Check sheet for the modelled part. Datum: model origin and axes. Units: mm. A direction names the side the tool comes from. Round coordinates to 2 decimals unless told otherwise and drop trailing zeros. Loops run counter-clockwise (first coordinate to the right, second up) from the corner with the lowest first, then second, coordinate; pieces in that order, holes last. Notation, with made-up numbers: M -36.5,-32 L 17.5,-32 A26 cw 17.5,-13 Z; hole C -34.75,-10 d9. An arc over 180 degrees is marked long. Write item = value, one per line. Start each with the question number.
(1) Cross-section at B-B on x = 0.55. Record the boundary of the cut face in (y, z).
(2) Set-up check for faces 5 (the face through (2, -5, -22)), 6 (the face through (4, 0, -18)): record each of +Z, -Z, +X, -X, +Y, -Y from which the full face is reachable in a straight line by a thin tool's end or side.
(3) Cross-section at D-D on x = 3.95. Record the boundary of the cut face in (y, z) (3 decimals).
(4) Cross-section at C-C on z = -11.5. Record the boundary of the cut face in (x, y).
(5) Cross-section at A-A on y = -7.25. Record the boundary of the cut face in (x, z).
(6) Go/stop test with flat-tipped pins: P1, Ø1, axis at x = 1, z = -5.5, coming from the +Y side; P2, Ø1.5, axis at x = 2.5, y = -8, coming from the +Z side; P3, Ø3, axis at x = 1.5, y = -10.5, coming from the +Z side; P4, Ø1.6, axis at x = 1, y = -3, coming from the +Z side. Record where each tip stops, or that it passes through.
(7) Mould release check, pull along Z, two halves, no side actions. Record for faces 1 (the face through (4, -19, 0)), 2 (the face through (3, -15, -30)), 3 (the face through (3.2, -13.3, -11.2)), 4 (the face through (4.6, -12.8, -11.5)): pulls with the +Z half, pulls with the -Z half, needs draft (parallel to the pull), parting line crosses it, or undercut.
(8) Scan lines: L1, parallel to Y at x = 4.7, z = -10 (3 decimals); L2, parallel to Z at x = 4.3, y = -12; L3, parallel to Z at x = 2.1, y = -7.5. Record each from-to range of solid material in increasing order. Write a range as from..to.
from build123d import *

# Parameters (mm, degrees)
SKETCH2_W               = 30
SKETCH2_H               = 30
SKETCH2_R               = 3.175
BOSS_EXTRUDE1_DEPTH     = 6
CUT_EXTRUDE1_DEPTH      = 43.848570571
CUT_EXTRUDE1_DEPTH_BACK = 3.2
SKETCH3_R               = 3.175


with BuildPart() as part:
    # Sketch2 → Boss-Extrude1 (new body)
    with BuildSketch(Plane(origin=(0, 0, 0), x_dir=(0, 0, -1), z_dir=(1, 0, 0))):
        with Locations((15, -15)):
            Rectangle(SKETCH2_W, SKETCH2_H)
        with Locations((10, -10)):
            Circle(SKETCH2_R, mode=Mode.SUBTRACT)
    extrude(amount=BOSS_EXTRUDE1_DEPTH)

    # Sketch3 → Cut-Extrude1 (cut, two sides: drawn at the far end of the back side and taken through both)
    with BuildSketch(Plane.ZY.offset(-CUT_EXTRUDE1_DEPTH_BACK)):
        with BuildLine():
            Line((-22, 0), (-22, -10))
            ThreePointArc((-22, -10), (-18.485281374, -18.485281374), (-10, -22))
            Line((-10, -22), (0, -22))
            Line((0, -22), (0, 0))
            Line((0, 0), (-22, 0))
        make_face()
        with Locations((-10, -10)):
            Circle(SKETCH3_R, mode=Mode.SUBTRACT)
    extrude(amount=CUT_EXTRUDE1_DEPTH + CUT_EXTRUDE1_DEPTH_BACK, mode=Mode.SUBTRACT)


solid = part.part
Result:
q1.outline = M -30,-30 L 0,-30 L 0,-22 L -10,-22 A12 cw -22,-10 L -22,0 L -30,0 Z
q2.face_5 = +Z, -X, +Y
q2.face_6 = +Z, -Z, +X, -X, +Y
q3.outline = M -30,-30 L 0,-30 L 0,0 L -30,0 Z; hole C -10,-10 d6.35
q4.outline = M 0,-30 L 6,-30 L 6,-12.8 L 3.2,-12.8 L 3.2,-21.91 L 0,-21.91 Z; M 3.2,-7.2 L 6,-7.2 L 6,0 L 3.2,0 Z
q5.outline = M 0,-30 L 6,-30 L 6,-11.59 L 3.2,-11.59 L 3.2,-22 L 0,-22 Z; M 3.2,-8.41 L 6,-8.41 L 6,0 L 3.2,0 Z
q6.P1 = -22
q6.P2 = 0
q6.P3 = -21.83
q6.P4 = -22
q7.face_1 = pulls with the +Z half
q7.face_2 = pulls with the -Z half
q7.face_3 = needs draft
q7.face_4 = undercut
q8.L1 = -30..-13.175, -6.825..0
q8.L2 = -30..-12.47, -7.53..0
q8.L3 = -30..-22
